```python
from build123d import *

# Parameters (mm, degrees)
SKETCH1_R           = 14
SKETCH1_R_2         = 10
BOSS_EXTRUDE1_DEPTH = 5
BOSS_EXTRUDE2_DEPTH = 5
CIRPATTERN1_COUNT   = 26


with BuildPart() as part:
    # Sketch1 → Boss-Extrude1 (new, symmetric)
    with BuildSketch(Plane.YZ):
        with Locations(Location((0, 0, 0), (0, 0, 270))):
            Circle(SKETCH1_R)
        with Locations(Location((0, 0, 0), (0, 0, 270))):
            Circle(SKETCH1_R_2, mode=Mode.SUBTRACT)
    extrude(amount=BOSS_EXTRUDE1_DEPTH, both=True)

    # Sketch1_3 → Boss-Extrude2 (add, symmetric)
    with BuildSketch(Plane.YZ):
        with BuildLine():
            Line((17, -0.6), (17, 0.6))
            Line((17, 0.6), (13.948476619, 1.2))
            ThreePointArc((13.948476619, 1.2), (13.987113224, 0.600552799), (14, 0))
            ThreePointArc((14, 0), (13.987113224, -0.600552799), (13.948476619, -1.2))
            Line((13.948476619, -1.2), (17, -0.6))
        make_face()
    boss_extrude2 = extrude(amount=BOSS_EXTRUDE2_DEPTH, both=True)

    # CirPattern1: Boss-Extrude2 ×26 about axis
    cirpattern1_axis = Axis((0, 0, 0), (1, 0, 0))
    for i in range(1, CIRPATTERN1_COUNT):
        add(boss_extrude2.rotate(cirpattern1_axis, i * 360 / CIRPATTERN1_COUNT))


solid = part.part
```
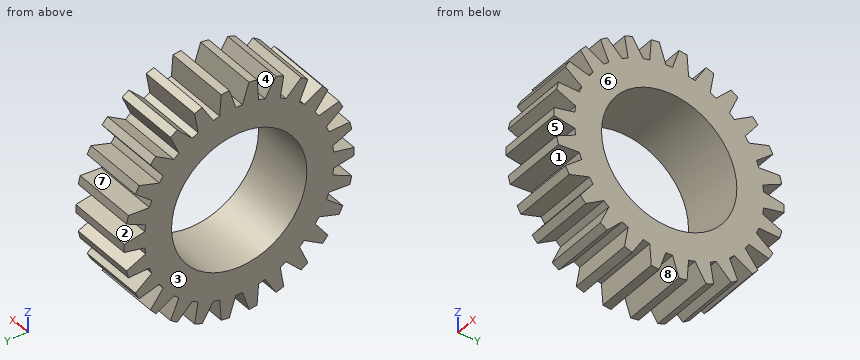
Can you work these out from the model? Positions are in its coordinate system, mm. Face numbers are marked on the shaded views. A direction names the side the tool comes from. Coordinates: 2 decimals unless noted, no trailing zeros. Loops run counter-clockwise (first coordinate to the right, second up) from the corner with the lowest first, then second, coordinate; pieces in that order, holes last.
1) I need wall thicknesses on probe 1 along Y at (x, z) = (-1.25, 0); probe 2 along Y at (x, z) = (3.75, 11.5); probe 3 along Y at (x, z) = (-3.25, 12.5). Which ranges of each line are inside material? Lowest first, please.
2) For pin 1 (2 mm diameter, centred on x = 2.5, y = 11.5, fed in from +Z); pin 2 (6 mm diameter, centred on x = 2, z = 5, fed in from +Y); pin 3 (4 mm diameter, centred on x = -3.5, y = 5.5, fed in from -Z), each with a flat end and sliding along its axis, tell me the tip position at first contact or that it passes through.
3) Which directions (+Z, -Z, +X, -X, +Y, -Y) give clear straight access to the entire face, cutting with the end or side of a thin tool? Please do the marked faces 4, 5, 6, 7 and 8.
4) Imagine slicing it at A-A on z = 0. List the corners of the cut face in (x, y) for me, plus the area to 3 significant figures.
5) Thinking about a two-plate mould opening in Y: for the marked faces 1, 2 and 3, which applies, pulls with the +Y half, pulls with the -Y half, needs draft (parallel to the pull), parting line crosses it, or undercut?
6) Imagine slicing it at C-C on z = -15. List the corners of the cut face in (x, y) for me.
7) Imagine slicing it at B-B on y = 0. List the corners of the cut face in (x, z) for me, plus the area to 3 significant figures.
Completed:
1. probe 1: y = -17 to -10, 10 to 17
1. probe 2: y = -12.52 to -11.95, -9.22 to 9.22, 11.95 to 12.52
1. probe 3: y = -9.65 to -7.28, -6.3 to 6.3, 7.28 to 9.65
2. pin 1: stops at z = 11.72
2. pin 2: stops at y = 16.65
2. pin 3: stops at z = -16.11
3. face 4: +Z, +X, -X
3. face 5: +X, -X, -Y
3. face 6: +Z, -Z, +X, +Y, -Y
3. face 7: +X, -X
3. face 8: -Z, +X, -X
4. outline: (-5, -17) - (5, -17) - (5, -10) - (-5, -10) - close; (-5, 10) - (5, 10) - (5, 17) - (-5, 17) - close
4. area: 140 mm2
5. face 1: undercut
5. face 2: pulls with the +Y half
5. face 3: needs draft
6. outline: (-5, -6.47) - (5, -6.47) - (5, -4.78) - (-5, -4.78) - close; (-5, -2.78) - (5, -2.78) - (5, -0.82) - (-5, -0.82) - close; (-5, 0.82) - (5, 0.82) - (5, 2.78) - (-5, 2.78) - close; (-5, 4.78) - (5, 4.78) - (5, 6.47) - (-5, 6.47) - close
7. outline: (-5, -14) - (5, -14) - (5, -10) - (-5, -10) - close; (-5, 10) - (5, 10) - (5, 14) - (-5, 14) - close
7. area: 80.0 mm2
